Geometry check sheet. Reference: the model listing, model coordinates, mm. Face numbers are marked on the shaded views. A direction names the side the tool comes from. Round coordinates to 2 decimals unless told otherwise and drop trailing zeros. Order: outer loops, then holes, each group sorted by start corner. A loop starts at its lowest first (then second) coordinate and runs counter-clockwise, first axis right, second up. Notation, with made-up numbers: M 47,-15.75 L 51,-15.75 A19 ccw 51,20.25 Z; hole C 43.5,7 d2. An arc over 180 degrees is marked long. Answer as a JSON object with one key per item and string values. Group by question number.
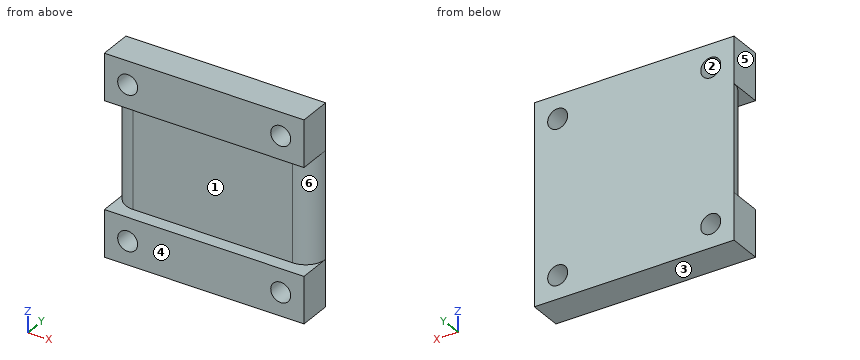
```python
from build123d import *

# Parameters (mm, degrees)
SKETCH1_W           = 30
SKETCH1_H           = 16
SKETCH1_H_2         = 7
SKETCH1_R           = 1.5
BOSS_EXTRUDE1_DEPTH = 5
SKETCH1_3_W         = 30
SKETCH1_3_H         = 16
CUT_EXTRUDE1_DEPTH  = 2
FILLET1_R           = 3


with BuildPart() as part:
    # Sketch1 → Boss-Extrude1 (new body)
    # profile 1 of 3: a face of its own
    with BuildSketch(Plane(origin=(0, 0, 0), x_dir=(1, 0, 0), z_dir=(0, 1, 0))):
        Rectangle(SKETCH1_W, SKETCH1_H)
    # profile 2 of 3: a face of its own
    with BuildSketch(Plane(origin=(0, 0, 0), x_dir=(1, 0, 0), z_dir=(0, 1, 0))):
        with Locations((0, 11.5)):
            Rectangle(SKETCH1_W, SKETCH1_H_2)
        with Locations(Location((-11.5, 11.5, 0), (0, 0, 270))):
            Circle(SKETCH1_R, mode=Mode.SUBTRACT)
        with Locations(Location((11.5, 11.5, 0), (0, 0, 270))):
            Circle(SKETCH1_R, mode=Mode.SUBTRACT)
    # profile 3 of 3: a face of its own
    with BuildSketch(Plane(origin=(0, 0, 0), x_dir=(1, 0, 0), z_dir=(0, 1, 0))):
        with Locations((0, -11.5)):
            Rectangle(SKETCH1_W, SKETCH1_H_2)
        with Locations(Location((-11.5, -11.5, 0), (0, 0, 270))):
            Circle(SKETCH1_R, mode=Mode.SUBTRACT)
        with Locations(Location((11.5, -11.5, 0), (0, 0, 270))):
            Circle(SKETCH1_R, mode=Mode.SUBTRACT)
    extrude(amount=BOSS_EXTRUDE1_DEPTH)

    # Sketch1<3> → Cut-Extrude1 (cut)
    with BuildSketch(Plane(origin=(0, 0, 0), x_dir=(1, 0, 0), z_dir=(0, 1, 0))):
        Rectangle(SKETCH1_3_W, SKETCH1_3_H)
    extrude(amount=CUT_EXTRUDE1_DEPTH, mode=Mode.SUBTRACT)

    # Fillet1
    fillet1_edges = [part.edges().sort_by_distance(p)[0] for p in [
        (15, 2, 0),
        (-15, 2, 0),
    ]]
    fillet(fillet1_edges, radius=FILLET1_R - 0.0001)  # a hair under: the kernel refuses the full size


solid = part.part
```
1) Sectioned sample at C-C (x = 11.5). Record the boundary of the cut face in (y, z).
2) Go/stop test with a flat-tipped pin: P1, Ø2.5, axis at x = 11.5, z = 11.5, coming from the -Y side. Record where the tip stops, or that it passes through.
3) Sectioned sample at D-D (y = 3.3). Record the boundary of the cut face in (x, z).
4) Sectioned sample at A-A (y = 0.6). Record the boundary of the cut face in (x, z), then the cut area to 3 significant figures.
5) Thickness scan on line 1 along X through (y, z) = (2.6, 11.5); line 2 along Z through (x, y) = (-5.25, 1.5); line 3 along X through (y, z) = (0.2, 12). Record the ranges inside material, lowest first. Write a range as [from, to].
6) Sectioned sample at B-B (z = 11.5). Record the boundary of the cut face in (x, y).
7) Release check for a two-part mould opening along Z. For the marked faces 1, 2, 3 and 4 record: +Z half, -Z half, draft (parallel to the pull), parting line (faces both ways), or undercut.
8) Set-up check for the marked faces 5 and 6: record each of +Z, -Z, +X, -X, +Y, -Y from which the full face is reachable in a straight line by a thin tool's end or side.
Final values:
{
 "1": {"outline": "M 0,-15 L 5,-15 L 5,-13 L 0,-13 Z; M 0,-10 L 5,-10 L 5,10 L 0,10 L 0,8 L 2,8 L 2,-8 L 0,-8 Z; M 0,13 L 5,13 L 5,15 L 0,15 Z"},
 "2": {"P1": "passes through"},
 "3": {"outline": "M -15,-15 L 15,-15 L 15,-8 L 14.47,-8 L 14.47,8 L 15,8 L 15,15 L -15,15 L -15,8 L -14.47,8 L -14.47,-8 L -15,-8 Z; hole C -11.5,-11.5 d3; hole C -11.5,11.5 d3; hole C 11.5,-11.5 d3; hole C 11.5,11.5 d3"},
 "4": {"outline": "M -15,-15 L 15,-15 L 15,-8 L -15,-8 Z; M -15,8 L 15,8 L 15,15 L -15,15 Z; hole C -11.5,-11.5 d3; hole C -11.5,11.5 d3; hole C 11.5,-11.5 d3; hole C 11.5,11.5 d3", "area": "392 mm^2"},
 "5": {"line 1": "x = [-15, -13], [-10, 10], [13, 15]", "line 2": "z = [-15, -8], [8, 15]", "line 3": "x = [-15, -12.91], [-10.09, 10.09], [12.91, 15]"},
 "6": {"outline": "M -15,0 L -13,0 L -13,5 L -15,5 Z; M -10,0 L 10,0 L 10,5 L -10,5 Z; M 13,0 L 15,0 L 15,5 L 13,5 Z"},
 "7": {"face 1": "undercut", "face 2": "undercut", "face 3": "-Z half", "face 4": "draft"},
 "8": {"face 5": "+Z, -Z, -X, +Y, -Y", "face 6": "+X, -Y"}
}
